Build history of the part. All positions in model axes, mm. A direction names the side the tool comes from. Give positions to 0.01 mm unless a question says otherwise; leave off trailing zeros. Loops run counter-clockwise (first coordinate to the right, second up) from the corner with the lowest first, then second, coordinate; pieces in that order, holes last.
1) Flat gauge pin, fed straight in: P1, Ø5.5, axis at y = -15.5, z = 46, coming from the +X side. Where does the tip first touch, or does it go through?
2) Wall check: line 1 (Y direction, x = -24, z = 30); line 2 (X direction, y = 12.5, z = 12.5); line 3 (Z direction, x = 1.5, y = -7). Give the ranges that are in metal, low to high.
3) Band-saw the part on D-D on z = 14. List the corners of the cut face in (x, y).
4) Band-saw the part on C-C on z = 30.5. List the corners of the cut face in (x, y), then the cut area to 3 significant figures.
5) Band-saw the part on A-A on x = 16. List the corners of the cut face in (y, z).
6) Band-saw the part on B-B on y = 0. List the corners of the cut face in (x, z), then the cut area to 3 significant figures.
7) Two-plate mould, pull along Y, no slides. Class faces 1 (the flat face through (-17, 25, 11)), 2 (the cylindrical face through (-25.271, -13.765, 14.772)), 3 (the flat face through (-25, 0, 51.5)): +Y half, -Y half, draft (parallel to the pull), parting line (faces both ways), or undercut.
8) 3-axis set-ups, long thin cutter, end or side, ignore diameter. For faces 4 (the flat face through (26.75, 0, 1)), 5 (the flat face through (2, 17, 2)), 6 (the flat face through (-20, -22, 8)): which of +Z, -Z, +X, -X, +Y, -Y reach the whole face in a straight line?
```python
from build123d import *

# Parameters (mm, degrees)
SKETCH2_W           = 53.5
SKETCH2_H           = 50
BOSS_EXTRUDE1_DEPTH = 51.5
SKETCH3_W           = 50.5
SKETCH3_H           = 50
CUT_EXTRUDE1_DEPTH  = 48.5
CHAMFER1_SIZE       = 14
CHAMFER1_SIZE2      = 19.269346887
SKETCH4_W           = 48.5
SKETCH4_H           = 44
CUT_EXTRUDE2_DEPTH  = 50.5
SKETCH5_R           = 1.75
SKETCH5_R_2         = 11.5
CUT_EXTRUDE3_DEPTH  = 10
CUT_EXTRUDE4_DEPTH  = 10
CHAMFER2_SIZE       = 5
FILLET1_R           = 2


with BuildPart() as part:
    # Sketch2 → Boss-Extrude1 (new body)
    with BuildSketch(Plane.XY):
        Rectangle(SKETCH2_W, SKETCH2_H)
    extrude(amount=BOSS_EXTRUDE1_DEPTH)

    # Sketch3 → Cut-Extrude1 (cut)
    with BuildSketch(Plane.XY.offset(51.5)):
        with Locations((1.5, 0)):
            Rectangle(SKETCH3_W, SKETCH3_H)
    extrude(amount=-CUT_EXTRUDE1_DEPTH, mode=Mode.SUBTRACT)

    # Chamfer1
    chamfer1_edges = [part.edges().sort_by_distance(p)[0] for p in [
        (-23.75, 0, 3),
    ]]
    chamfer1_side = [part.faces().sort_by_distance(p)[0] for p in [
        (1.5, 0, 3),
    ]]
    chamfer(chamfer1_edges, length=CHAMFER1_SIZE, length2=CHAMFER1_SIZE2, reference=chamfer1_side[0])

    # Sketch4 → Cut-Extrude2 (cut)
    with BuildSketch(Plane(origin=(26.75, 0, 0), x_dir=(0, 0, -1), z_dir=(1, 0, 0))):
        with Locations((-27.25, 0)):
            Rectangle(SKETCH4_W, SKETCH4_H)
    extrude(amount=-CUT_EXTRUDE2_DEPTH, mode=Mode.SUBTRACT)

    # Sketch5 → Cut-Extrude3 (cut)
    with BuildSketch(Plane.ZY.offset(26.75)):
        with Locations((46, 15.5)):
            Circle(SKETCH5_R)
        with Locations((46, -15.5)):
            Circle(SKETCH5_R)
        with Locations((15, 15.5)):
            Circle(SKETCH5_R)
        with Locations((15, -15.5)):
            Circle(SKETCH5_R)
        with Locations((30.5, 0)):
            Circle(SKETCH5_R_2)
    extrude(amount=-CUT_EXTRUDE3_DEPTH, mode=Mode.SUBTRACT)

    # Sketch6 → Cut-Extrude4 (cut)
    with BuildSketch(Plane.XY.offset(3)):
        with BuildLine():
            Line((-13.25, 17), (16.75, 17))
            ThreePointArc((16.75, 17), (18.75, 15), (16.75, 13))
            Line((16.75, 13), (-13.25, 13))
            ThreePointArc((-13.25, 13), (-15.25, 15), (-13.25, 17))
        make_face()
        with BuildLine():
            Line((-13.25, -13), (16.75, -13))
            ThreePointArc((16.75, -13), (18.75, -15), (16.75, -17))
            Line((16.75, -17), (-13.25, -17))
            ThreePointArc((-13.25, -17), (-15.25, -15), (-13.25, -13))
        make_face()
    extrude(amount=-CUT_EXTRUDE4_DEPTH, mode=Mode.SUBTRACT)

    # Chamfer2
    chamfer2_edges = [part.edges().sort_by_distance(p)[0] for p in [
        (-25.25, -25, 51.5),
        (-25.25, 25, 51.5),
        (26.75, -25, 1.5),
        (26.75, 25, 1.5),
    ]]
    chamfer(chamfer2_edges, length=CHAMFER2_SIZE)

    # Fillet1
    fillet1_edges = [part.edges().sort_by_distance(p)[0] for p in [
        (-23.75, 0, 3),
        (-26.75, 0, 0),
    ]]
    fillet(fillet1_edges, radius=FILLET1_R)


solid = part.part
```
Findings below:
1. P1: stops at x = -23.75
2. line 1: y = -25 to -11.49, 11.49 to 25
2. line 2: x = -26.75 to -23.75
2. line 3: z = 0 to 3
3. outline: (-26.75, -25) - (-17.74, -25) - (-17.74, -22) - (-23.75, -22) - (-23.75, -16.94) - (-26.75, -16.94) - close; (-26.75, -14.06) - (-23.75, -14.06) - (-23.75, 14.06) - (-26.75, 14.06) - close; (-26.75, 16.94) - (-23.75, 16.94) - (-23.75, 22) - (-17.74, 22) - (-17.74, 25) - (-26.75, 25) - close
4. outline: (-26.75, -25) - (-23.75, -25) - (-23.75, -11.5) - (-26.75, -11.5) - close; (-26.75, 11.5) - (-23.75, 11.5) - (-23.75, 25) - (-26.75, 25) - close
4. area: 81.0 mm2
5. outline: (-25, 0) - (-17, 0) - (-17, 3) - (-25, 3) - close; (-13, 0) - (13, 0) - (13, 3) - (-13, 3) - close; (17, 0) - (25, 0) - (25, 3) - (17, 3) - close
6. outline: (-26.75, 2) arc R2 ccw to (-24.75, 0) - (26.75, 0) - (26.75, 3) - (-21.75, 3) arc R2 cw to (-23.75, 5) - (-23.75, 19) - (-26.75, 19) - close; (-26.75, 42) - (-23.75, 42) - (-23.75, 51.5) - (-26.75, 51.5) - close
6. area: 237 mm2
7. face 1: +Y half
7. face 2: undercut
7. face 3: draft
8. face 4: +Z, -Z, +X, +Y, -Y
8. face 5: +Z, -Z
8. face 6: +Z, +X
